Answer from the drawing. Dimensions are ordinates in mm from the lowest x, y and z of the part. Give positions to 0.01 mm unless a question says otherwise; leave off trailing zeros. Write each loop counter-clockwise with the first axis right and the second up, starting at its lowest first coordinate (ties: lowest second). Pieces come first, ordered by that corner, then holes. Notation, with made-up numbers: M 52,85.5 L 86,85.5 A29 ccw 86,106.5 Z; hole C 21.5,-19 d5. An arc over 180 degrees is marked long. Answer as a JSON object with one key per item and string values.
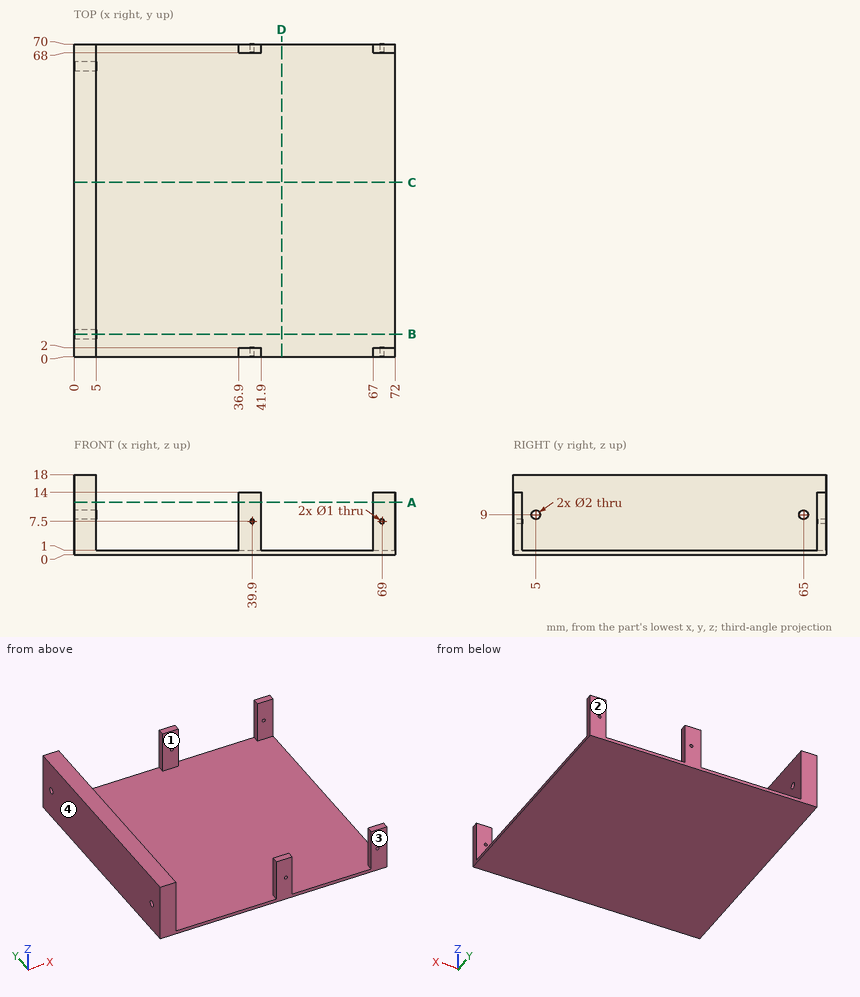
1. Consider line 1 along Y through (x, z) = (68.5, 4.5); line 2 along Z through (x, y) = (69, 0.4); line 3 along X through (y, z) = (10, 1.75). Determine where each line is inside the solid, lowest interval first.
Verdict:
{"line 1": "y = 0 to 2, 68 to 70", "line 2": "z = 0 to 7, 8 to 14", "line 3": "x = 0 to 5"}
2. A cutting plane is placed at B-B, the plane y = 5. Give the vertices of the cut face in (x, z), plus the area to 3 significant figures.
Verdict:
{"outline": "M 0,0 L 72,0 L 72,1 L 5,1 L 5,8 L 0,8 Z; M 0,10 L 5,10 L 5,18 L 0,18 Z", "area": "147 mm2"}
3. The mould has two halves that part along Y. Classify the marked faces 1, 2, 3 and 4: released by +Y, released by -Y, zero draft, split by the parting line, or undercut.
Verdict:
{"face 1": "undercut", "face 2": "released by +Y", "face 3": "released by -Y", "face 4": "zero draft"}
4. A cutting plane is placed at D-D, the plane x = 46.5. Give the vertices of the cut face in (y, z), plus the area to 3 significant figures.
Verdict:
{"outline": "M 0,0 L 70,0 L 70,1 L 0,1 Z", "area": "70.0 mm2"}
5. Flat-ended cylindrical pins translate along their axes: pin 1 (1.6 mm diameter, centred on x = 70, y = 69, fed in from +Z); pin 2 (12 mm diameter, centred on x = 32.5, y = 20, fed in from +Z); pin 3 (2.5 mm diameter, centred on y = 65, z = 9, fed in from +X). Find the tip coordinate at first contact, or state that the pin passes through.
Verdict:
{"pin 1": "stops at z = 14", "pin 2": "stops at z = 1", "pin 3": "stops at x = 5"}
6. A cutting plane is placed at A-A, the plane z = 11.75. Give the vertices of the cut face in (x, y).
Verdict:
{"outline": "M 0,0 L 5,0 L 5,70 L 0,70 Z; M 36.9,0 L 41.9,0 L 41.9,2 L 36.9,2 Z; M 36.9,68 L 41.9,68 L 41.9,70 L 36.9,70 Z; M 67,0 L 72,0 L 72,2 L 67,2 Z; M 67,68 L 72,68 L 72,70 L 67,70 Z"}
7. A cutting plane is placed at C-C, the plane y = 39. Give the vertices of the cut face in (x, z).
Verdict:
{"outline": "M 0,0 L 72,0 L 72,1 L 5,1 L 5,18 L 0,18 Z"}
